from build123d import *

# Parameters (mm, degrees)
F0_W     = 101.6
F0_H     = 50.8
F1_DEPTH = 113.03
F2_DEPTH = 6.35
F3_W     = 11.43
F3_H     = 3.175
F4_DEPTH = 63.5
F5_W     = 2.286
F5_H     = 3.175
F6_DEPTH = 63.5
F7_W     = 10.16
F7_H     = 43.18
F8_DEPTH = 73.66


# Not quite as in the source:
# - a feature names something its author has since deleted; it is built from what else it names


with BuildPart() as f1:
    # F0 (on Top) → F1 (new body)
    with BuildSketch(Plane.XY):
        with BuildLine():
            ThreePointArc((53.34, 25.4), (52.5960512242, 27.1960512242), (50.8, 27.94))
            Line((50.8, 27.94), (-50.8, 27.94))
            ThreePointArc((-50.8, 27.94), (-52.5960512242, 27.1960512242), (-53.34, 25.4))
            Line((-53.34, 25.4), (-53.34, -25.4))
            ThreePointArc((-53.34, -25.4), (-52.5960512242, -27.1960512242), (-50.8, -27.94))
            Line((-50.8, -27.94), (50.8, -27.94))
            ThreePointArc((50.8, -27.94), (52.5960512242, -27.1960512242), (53.34, -25.4))
            Line((53.34, -25.4), (53.34, 25.4))
        make_face()
        Rectangle(F0_W, F0_H, mode=Mode.SUBTRACT)
    extrude(amount=F1_DEPTH)

    # F0 (on Top) → F2 (join)
    with BuildSketch(Plane.XY):
        with BuildLine():
            ThreePointArc((53.34, 25.4), (52.5960512242, 27.1960512242), (50.8, 27.94))
            Line((50.8, 27.94), (-50.8, 27.94))
            ThreePointArc((-50.8, 27.94), (-52.5960512242, 27.1960512242), (-53.34, 25.4))
            Line((-53.34, 25.4), (-53.34, -25.4))
            ThreePointArc((-53.34, -25.4), (-52.5960512242, -27.1960512242), (-50.8, -27.94))
            Line((-50.8, -27.94), (50.8, -27.94))
            ThreePointArc((50.8, -27.94), (52.5960512242, -27.1960512242), (53.34, -25.4))
            Line((53.34, -25.4), (53.34, 25.4))
        make_face()
        Rectangle(F0_W, F0_H, mode=Mode.SUBTRACT)
        Rectangle(F0_W, F0_H)
    extrude(amount=F2_DEPTH)

    # F3 (on face) → F4 (join)
    with BuildSketch(Plane.XY.offset(6.35)):
        with Locations((-45.085, 0.1905)):
            Rectangle(F3_W, F3_H)
    extrude(amount=F4_DEPTH)

    # F5 (on face) → F6 (join)
    with BuildSketch(Plane.XY.offset(6.35)):
        with Locations((49.657, 5.3975)):
            Rectangle(F5_W, F5_H)
        with Locations((49.657, 0.1905)):
            Rectangle(F5_W, F5_H)
    extrude(amount=F6_DEPTH)

    # F7 (on Right) → F8 (cut)
    with BuildSketch(Plane.YZ):
        with Locations((5.08, 55.372)):
            Rectangle(F7_W, F7_H)
    extrude(amount=-F8_DEPTH, mode=Mode.SUBTRACT)


solid = f1.part
Read the model definition and answer for the solid it produces. Units are mm, in the model's axes. A direction names the side the tool comes from. Round coordinates to 2 decimals unless told otherwise and drop trailing zeros. Order: outer loops, then holes, each group sorted by start corner. A loop starts at its lowest first (then second) coordinate and runs counter-clockwise, first axis right, second up.
1) The part is cut by section B-B on y = 12. Write down the section's boundary in (x, z).
2) The part is cut by section C-C on x = 18.5. Write down the section's boundary in (y, z), plus the area to 3 significant figures.
3) The part is cut by section A-A on z = 27. Write down the section's boundary in (x, y) (3 decimals).
4) The part is cut by section D-D on z = 73. Write down the section's boundary in (x, y).
5) The mould has two halves that part along Y. Classify faces 4 (the face through (52.616, 27.176, 55.724)), 5 (the face through (-45, 1.778, 20)), 6 (the face through (-1, -27.94, 56)), 7 (the face through (-4, -27, 113.03)): released by +Y, released by -Y, zero draft, split by the parting line, or undercut.
6) Flat-ended cylindrical pins translate along their axes: pin 1 (3.5 mm diameter, centred on y = 5, z = 38, fed in from -X); pin 2 (1.5 mm diameter, centred on x = -43, y = -0.5, fed in from +Z); pin 3 (2 mm diameter, centred on x = 34, y = -16.5, fed in from +Z). Find the tip coordinate at first contact, or state that the pin passes through.
7) For faces 1 (the face through (-50.8, -6, 59)), 2 (the face through (-46, 0, 55)), 3 (the face through (1, 27.94, 56)), determine the directions among +Z, -Z, +X, -X, +Y, -Y from which every point of the face is accessible in a straight line to the end or side of a thin tool.
8) Straight lines are drawn through the part: L1, parallel to Y at x = 20.5, z = 51; L2, parallel to X at y = 2, z = 23; L3, parallel to X at y = -0.5, z = 62.5. For each, find the intervals that lie inside material, in ascending order.
Resolved:
1. outline: (-53.34, 0) - (53.34, 0) - (53.34, 113.03) - (50.8, 113.03) - (50.8, 6.35) - (-50.8, 6.35) - (-50.8, 113.03) - (-53.34, 113.03) - close
2. outline: (-27.94, 0) - (27.94, 0) - (27.94, 113.03) - (25.4, 113.03) - (25.4, 6.35) - (-25.4, 6.35) - (-25.4, 113.03) - (-27.94, 113.03) - close
2. area: 897 mm2
3. outline: (-53.34, -25.4) arc R2.54 ccw to (-50.8, -27.94) - (50.8, -27.94) arc R2.54 ccw to (53.34, -25.4) - (53.34, 25.4) arc R2.54 ccw to (50.8, 27.94) - (-50.8, 27.94) arc R2.54 ccw to (-53.34, 25.4) - close; hole (-50.8, -25.4) - (50.8, -25.4) - (50.8, -1.397) - (48.514, -1.397) - (48.514, 1.778) - (50.8, 1.778) - (50.8, 3.81) - (48.514, 3.81) - (48.514, 6.985) - (50.8, 6.985) - (50.8, 25.4) - (-50.8, 25.4) - (-50.8, 1.778) - (-39.37, 1.778) - (-39.37, -1.397) - (-50.8, -1.397) - close
4. outline: (-53.34, -25.4) arc R2.54 ccw to (-50.8, -27.94) - (50.8, -27.94) arc R2.54 ccw to (53.34, -25.4) - (53.34, 25.4) arc R2.54 ccw to (50.8, 27.94) - (-50.8, 27.94) arc R2.54 ccw to (-53.34, 25.4) - (-53.34, 10.16) - (-50.8, 10.16) - (-50.8, 25.4) - (50.8, 25.4) - (50.8, -25.4) - (-50.8, -25.4) - (-50.8, 0) - (-53.34, 0) - close
5. face 4: released by +Y
5. face 5: undercut
5. face 6: released by -Y
5. face 7: zero draft
6. pin 1: stops at x = 48.51
6. pin 2: stops at z = 69.85
6. pin 3: stops at z = 6.35
7. face 1: +Z
7. face 2: -X
7. face 3: +Z, -Z, +X, -X, +Y
8. L1: y = -27.94 to -25.4, 25.4 to 27.94
8. L2: x = -53.34 to -50.8, 50.8 to 53.34
8. L3: x = -53.34 to -39.37, 48.51 to 53.34
